Geometry check sheet. Reference: the model listing, model coordinates, mm. Round coordinates to 2 decimals unless told otherwise and drop trailing zeros. Order: outer loops, then holes, each group sorted by start corner. A loop starts at its lowest first (then second) coordinate and runs counter-clockwise, first axis right, second up.
(1) Sectioned sample at A-A (x = 0). Record the boundary of the cut face in (y, z), plus the area to 3 significant figures.
(2) Release check for a two-part mould opening along X. For faces 1 (the face through (16, -95, -21)), 2 (the face through (-23.846, 1.316, 7.509)), 3 (the face through (6.94, -1.32, -31.24)) record: +X half, -X half, draft (parallel to the pull), parting line (faces both ways), or undercut.
(3) Sectioned sample at C-C (y = -8). Record the boundary of the cut face in (x, z), plus the area to 3 significant figures.
(4) Material ranges on line 1 along Z through (x, y) = (0, -48.5); line 2 along X through (y, z) = (25, 1); line 3 along Z through (x, y) = (-9.5, 32), recorded low to high.
(5) Sectioned sample at B-B (z = 0). Record the boundary of the cut face in (x, y), plus the area to 3 significant figures.
(6) Go/stop test with flat-tipped pins: pin 1 (2 mm diameter, centred on x = -15, y = 43, fed in from +Z) (3 decimals); pin 2 (6 mm diameter, centred on y = 11, z = 19.5, fed in from -X); pin 3 (1 mm diameter, centred on x = -20, y = -58, fed in from +Z). Record where each tip stops, or that it passes through.
from build123d import *

# Parameters (mm, degrees)
F0_W    = 7
F0_H    = 95
F2_SIZE = 1
F3_SIZE = 1
F4_SIZE = 1


with BuildPart() as f1:
    # F0 (on Top) → F1 (revolve)
    with BuildSketch(Plane.XY):
        with Locations((-28.5, -47.5)):
            Rectangle(F0_W, F0_H)
        with Locations((-28.5, 47.5)):
            Rectangle(F0_W, F0_H)
    revolve(axis=Axis((0, 0, 0), (0, 1, 0)))

    # F2
    f2_edges = [f1.edges().sort_by_distance(p)[0] for p in [
        (25, -95, 0),
        (-25, 0, 0),
        (25, 95, 0),
    ]]
    chamfer(f2_edges, length=F2_SIZE)

    # F3
    f3_edges = [f1.edges().sort_by_distance(p)[0] for p in [
        (32, -95, 0),
    ]]
    chamfer(f3_edges, length=F3_SIZE)

    # F4
    f4_edges = [f1.edges().sort_by_distance(p)[0] for p in [
        (32, 95, 0),
    ]]
    chamfer(f4_edges, length=F4_SIZE)


solid = f1.part
Answer below:
1. outline: (-95, -31) - (-94, -32) - (94, -32) - (95, -31) - (95, -26) - (94, -25) - (-94, -25) - (-95, -26) - close; (-95, 26) - (-94, 25) - (94, 25) - (95, 26) - (95, 31) - (94, 32) - (-94, 32) - (-95, 31) - close
1. area: 2,660 mm2
2. face 1: draft
2. face 2: undercut
2. face 3: parting line
3. outline: circle Ø64 at (0, 0); hole circle Ø50 at (0, 0)
3. area: 1,250 mm2
4. line 1: z = -32 to -25, 25 to 32
4. line 2: x = -31.98 to -24.98, 24.98 to 31.98
4. line 3: z = -30.56 to -23.12, 23.12 to 30.56
5. outline: (-32, -94) - (-31, -95) - (-26, -95) - (-25, -94) - (-25, 94) - (-26, 95) - (-31, 95) - (-32, 94) - close; (25, -94) - (26, -95) - (31, -95) - (32, -94) - (32, 94) - (31, 95) - (26, 95) - (25, 94) - close
5. area: 2,660 mm2
6. pin 1: stops at z = 28.775
6. pin 2: stops at x = -27.42
6. pin 3: stops at z = 25.37
